Geometry: final body of the model. Coordinates: model frame, mm. Face numbers are marked on the shaded views. Give positions to 0.01 mm unless a question says otherwise; leave off trailing zeros. Write each loop counter-clockwise with the first axis right and the second up, starting at its lowest first coordinate (ties: lowest second). Pieces come first, ordered by that corner, then holes. Notation, with made-up numbers: (61.25, -27) -> (106.25, -27) arc R19 cw to (106.25, -15) -> close; hole circle Ø7 at (10.25, -38.75). An arc over 180 degrees is marked (long way). Answer as a JSON object with one key per item and string values.
from build123d import *

# Parameters (mm, degrees)
SKETCH1_R           = 25.4
BOSS_EXTRUDE1_DEPTH = 10.16
SKETCH2_R           = 4.7625
CUT_EXTRUDE1_DEPTH  = 38.33022368
SKETCH3_W           = 1.768395793
SKETCH3_H           = 3.093534736
CUT_EXTRUDE2_DEPTH  = 38.33022368


with BuildPart() as part:
    # Sketch1 → Boss-Extrude1 (new body)
    with BuildSketch(Plane.YZ):
        with Locations(Location((0, 0, 0), (0, 0, 270))):
            Circle(SKETCH1_R)
    extrude(amount=BOSS_EXTRUDE1_DEPTH)

    # Sketch2 → Cut-Extrude1 (cut, through all)
    with BuildSketch(Plane.YZ):
        with Locations(Location((5.08, 0, 0), (0, 0, 270))):
            Circle(SKETCH2_R)
    extrude(amount=CUT_EXTRUDE1_DEPTH, mode=Mode.SUBTRACT)

    # Sketch3 → Cut-Extrude2 (cut, through all)
    with BuildSketch(Plane.YZ):
        with Locations((10.482302104, -0.040732632)):
            Rectangle(SKETCH3_W, SKETCH3_H)
    extrude(amount=CUT_EXTRUDE2_DEPTH, mode=Mode.SUBTRACT)


solid = part.part
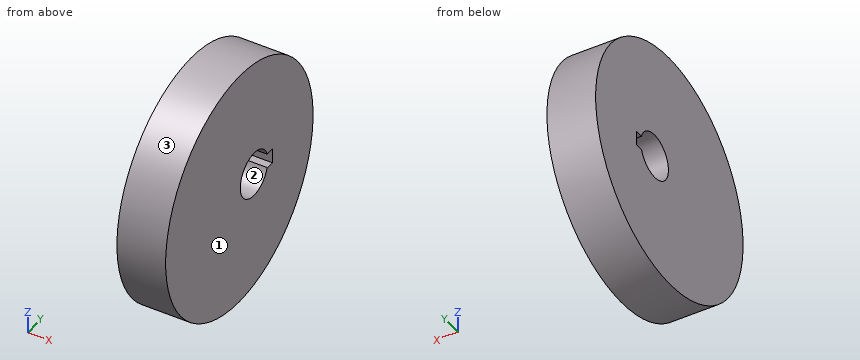
Q1. Mould query, pull axis Y, two halves, no side actions, for the marked faces 1, 2 and 3. Classes: pulls with the +Y half, pulls with the -Y half, needs draft (parallel to the pull), parting line crosses it, or undercut.
Values:
{"face 1": "needs draft", "face 2": "undercut", "face 3": "parting line crosses it"}
Q2. Material intervals for L1, parallel to Y at x = 7.5, z = 0; L2, parallel to Z at x = 2.75, y = 5.08; L3, parallel to Y at x = 5.5, z = -9, sorted ascending. Write a range as from..to.
Values:
{"L1": "-25.4..0.32, 11.37..25.4", "L2": "-24.89..-4.76, 4.76..24.89", "L3": "-23.75..23.75"}
Q3. First-contact query: P1, Ø3, axis at x = 2, z = -11, coming from the +Y side; P2, Ø3.5, axis at x = 4.5, z = -1, coming from the -Y side; P3, Ø7.5, axis at y = 5.08, z = 0, coming from the +X side; P4, Ø1.9, axis at x = 4, y = 10.5, coming from the -Z side. Flat tips, straight axial feed; report the tip coordinate or a pass-through.
Values:
{"P1": "y = 23.56", "P2": "y = -25.4", "P3": "through", "P4": "z = -23.54"}
Q4. Cut plane B-B (y = 9). Return the cut outline in (x, z), and give its area (3 significant figures).
Values:
{"outline": "(0, -23.75) -> (10.16, -23.75) -> (10.16, -2.7) -> (0, -2.7) -> close; (0, 2.7) -> (10.16, 2.7) -> (10.16, 23.75) -> (0, 23.75) -> close", "area": "428 mm²"}
Q5. Cut plane A-A (z = 0). Return the cut outline in (x, y), and give its area (3 significant figures).
Values:
{"outline": "(0, -25.4) -> (10.16, -25.4) -> (10.16, 0.32) -> (0, 0.32) -> close; (0, 11.37) -> (10.16, 11.37) -> (10.16, 25.4) -> (0, 25.4) -> close", "area": "404 mm²"}
Q6. Cut plane D-D (y = -16). Return the cut outline in (x, z), and give its area (3 significant figures).
Values:
{"outline": "(0, -19.73) -> (10.16, -19.73) -> (10.16, 19.73) -> (0, 19.73) -> close", "area": "401 mm²"}
